Autodesk Inventor part; units mm, degrees
ref_plane "YZ Plane" through (0, 0, 0) normal (1, 0, 0) x (0, 1, 0)
ref_plane "XZ Plane" through (0, 0, 0) normal (0, 1, 0) x (-1, 0, 0)
ref_plane "XY Plane" through (0, 0, 0) normal (0, 0, 1) x (1, 0, 0)
sketch "Boceto1" plane through (0, 0, 0) normal (0, 1, 0) x (-1, 0, 0)
  line L0 (-97.5, 97.5) -> (97.5, 97.5)
  line L1 (97.5, 97.5) -> (97.5, -97.5)
  line L2 (97.5, -97.5) -> (-97.5, -97.5)
  line L3 (-97.5, -97.5) -> (-97.5, 97.5)
  line L4 (-97.5, 97.5) -> (97.5, -97.5) construction
  line L5 (97.5, 97.5) -> (-97.5, -97.5) construction
  point P0 (0, 0)
  dimension "d0" = 195
  dimension "d1" = 195
extrude "Extrusión1" add sketch "Boceto1" along normal mid plane 4.4
sketch "Boceto4" plane through (0, -2.2, 0) normal (0, -1, 0) x (1, 0, 0)
  line L0 (97.5, -97.5) -> (97.5, 97.5) construction
  line L1 (-97.5, 97.5) -> (-97.5, -97.5) construction
  line L2 (84.1, -93.1) -> (-84.1, -93.1)
  line L3 (-84.1, -93.1) -> (-84.1, -84.1)
  line L4 (-84.1, -84.1) -> (84.1, -84.1)
  line L5 (84.1, -84.1) -> (84.1, -93.1)
  line L6 (-97.5, -97.5) -> (97.5, -97.5) construction
  line L7 (93.1, -84.1) -> (84.1, -84.1)
  line L8 (84.1, -84.1) -> (84.1, 84.1)
  line L9 (84.1, 84.1) -> (93.1, 84.1)
  line L10 (93.1, 84.1) -> (93.1, -84.1)
  line L11 (0, -126.8945) -> (0, 107.949)
  line L12 (-84.1, -84.1) -> (-84.1, 84.1)
  line L13 (-84.1, 84.1) -> (-93.1, 84.1)
  line L14 (-93.1, 84.1) -> (-93.1, -84.1)
  line L15 (-93.1, -84.1) -> (-84.1, -84.1)
  line L16 (84.1, 84.1) -> (-84.1, 84.1)
  line L17 (84.1, 93.1) -> (-84.1, 93.1)
  line L18 (84.1, 84.1) -> (84.1, 93.1)
  line L19 (-84.1, 84.1) -> (-84.1, 93.1)
  point P0 (0, 0)
  point P1 (-84.1, -88.6)
  point P2 (88.6, -84.1)
  point P3 (84.1, -84.1)
  point P4 (84.1, -84.1)
  point P5 (84.1, -84.1)
  point P6 (84.1, -84.1)
  point P7 (-84.1, 84.1)
  point P8 (-84.1, 84.1)
  point P9 (-84.1, 84.1)
  point P10 (-84.1, 84.1)
  dimension "d20" = 4.4
  dimension "d21" = 9
  dimension "d22" = 13.4
  dimension "d23" = 13.4
  dimension "d24" = 4.4
  dimension "d25" = 9
  dimension "d26" = 13.4
  dimension "d30" = 9
extrude "Extrusión6" add sketch "Boceto4" along normal blind 9 contours L2 L11 L4 L5 | L2 L3 L4 L11 | L8 L9 L10 L7 | L16 L11 L17 L18 | L15 L14 L13 L12 | L16 L19 L17 L11
sketch "Boceto5" plane through (0, -11.2, 0) normal (0, -1, 0) x (1, 0, 0)
  line L0 (-84.1, -93.1) -> (84.1, -93.1) construction
  line L1 (93.1, -84.1) -> (93.1, 84.1) construction
  line L2 (-93.1, 84.1) -> (-93.1, -84.1) construction
  line L3 (84.1, 93.1) -> (-84.1, 93.1) construction
  line L4 (84.1, -93.1) -> (-84.1, -93.1)
  line L5 (-93.1, -84.1) -> (-93.1, 84.1)
  line L6 (-84.1, 93.1) -> (84.1, 93.1)
  line L7 (93.1, 84.1) -> (93.1, -84.1)
  line L8 (84.1, -93.1) -> (84.1, -84.1)
  line L9 (84.1, -84.1) -> (-84.1, -84.1) construction
  line L10 (84.1, -93.1) -> (84.1, -84.1)
  line L11 (84.1, -84.1) -> (93.1, -84.1)
  line L12 (93.1, 84.1) -> (84.1, 84.1)
  line L13 (84.1, 84.1) -> (84.1, 93.1)
  line L14 (-93.1, 84.1) -> (-84.1, 84.1)
  line L15 (-84.1, 84.1) -> (-84.1, 93.1)
  line L16 (-93.1, -84.1) -> (-84.1, -84.1)
  line L17 (-84.1, -93.1) -> (-84.1, -84.1)
  line L18 (-84.1, -84.1) -> (-93.1, -84.1)
  point P0 (0, 0)
extrude "Extrusión7" add sketch "Boceto5" along normal blind 1.65
sketch "Boceto6" plane through (0, -12.85, 0) normal (0, -1, 0) x (1, 0, 0)
  line L0 (-84.1, -84.1) -> (84.1, -84.1) construction
  line L1 (53.1, -84.1) -> (43.1, -84.1)
  line L2 (43.1, -84.1) -> (43.1, -64.1)
  line L3 (43.1, -64.1) -> (53.1, -64.1)
  line L4 (53.1, -64.1) -> (53.1, -84.1)
  line L5 (93.1, -84.1) -> (93.1, 84.1)
  line L6 (84.1, -84.1) -> (84.1, 84.1)
  line L7 (64.1, -53.1) -> (84.1, -53.1)
  line L8 (84.1, -53.1) -> (84.1, -43.1)
  line L9 (84.1, -43.1) -> (64.1, -43.1)
  line L10 (64.1, -43.1) -> (64.1, -53.1)
  line L11 (-84.1, -93.1) -> (84.1, -93.1)
  point P0 (0, 0)
  dimension "d35" = 40
  dimension "d36" = 10
  dimension "d37" = 20
  dimension "d38" = 40
  dimension "d39" = 10
  dimension "d40" = 20
extrude "Extrusión8" add sketch "Boceto6" along normal blind 15
sketch "Boceto7" plane through (43.1, -12.85, -84.1) normal (-1, 0, 0) x (0, 0, 1)
  line L0 (0, 0) -> (20, 0)
  line L1 (0, 0) -> (0, -15) construction
  line L2 (20, -15) -> (0, -15) construction
  line L3 (20, 0) -> (20, -15) construction
  line L4 (0, 0) -> (20, 0)
  circle A0 centre (10, -7.5) radius 3.85
  point P0 (84.1, 12.85)
  dimension "d43" = 7.7
extrude "Extrusión9" add sketch "Boceto7" along normal blind 4
sketch "Boceto8" plane through (39.1, -20.35, -74.1) normal (-1, 0, 0) x (0, 0, 1)
  circle A0 centre (0, 0) radius 3.85
  circle A1 centre (0, 0) radius 7.25
  point P0 (74.1, 20.35)
  dimension "d46" = 14.5
extrude "Extrusión10" add sketch "Boceto8" along normal up to surface (39.1 mm away)
sketch "Boceto10" plane through (39.1, -20.35, -74.1) normal (-1, 0, 0) x (0, 0, 1)
  circle A0 centre (0, 0) radius 3.85
  point P0 (74.1, 20.35)
extrude "Extrusión11" add sketch "Boceto10" along normal up to surface (39.1 mm away)
mirror "Simetría4" about plane through (0, 0, 0) normal (1, 0, 0) of "Extrusión9", "Extrusión10", "Extrusión11", "Extrusión8"
sketch "Boceto11" plane through (-84.1, -27.85, -53.1) normal (0, -1, 0) x (1, 0, 0)
  line L0 (20, 0) -> (0, 0)
  line L1 (20, 10) -> (20, 0)
  line L2 (0, 10) -> (20, 10)
  line L3 (0, 0) -> (0, 10)
  point P0 (84.1, 53.1)
extrude "Extrusión12" cut sketch "Boceto11" against normal up to surface (15 mm away)
sketch "Boceto12" plane through (64.1, -12.85, -43.1) normal (0, 0, 1) x (1, 0, 0)
  line L0 (0, 0) -> (20, 0)
  line L1 (0, 0) -> (0, -15)
  line L2 (20, -15) -> (0, -15)
  line L3 (20, 0) -> (20, -15)
  circle A0 centre (10, -7.5) radius 3.85
  point P0 (-64.1, 12.85)
  dimension "d53" = 7.7
extrude "Extrusión13" add sketch "Boceto12" along normal blind 4 contours A0
sketch "Boceto13" plane through (74.1, -20.35, -39.1) normal (0, 0, 1) x (1, 0, 0)
  circle A0 centre (0, 0) radius 3.85
  circle A1 centre (0, 0) radius 7.25
  point P0 (-74.1, 20.35)
  dimension "d56" = 14.5
extrude "Extrusión14" add sketch "Boceto13" along normal up to surface (39.1 mm away)
sketch "Boceto14" plane through (74.1, -20.35, -39.1) normal (0, 0, 1) x (1, 0, 0)
  circle A0 centre (0, 0) radius 3.85
  point P0 (-74.1, 20.35)
extrude "Extrusión15" add sketch "Boceto14" along normal up to surface (39.1 mm away)
mirror "Simetría5" about plane through (0, 0, 0) normal (0, 0, 1) of "Extrusión15", "Extrusión14", "Extrusión13", "Extrusión12", "Extrusión8"
sketch "Boceto15" plane through (43.1, -27.85, 64.1) normal (0, -1, 0) x (1, 0, 0)
  line L0 (10, 0) -> (0, 0)
  line L1 (10, 20) -> (10, 0)
  line L2 (0, 20) -> (10, 20)
  line L3 (0, 0) -> (0, 20)
  point P0 (-43.1, -64.1)
extrude "Extrusión16" cut sketch "Boceto15" against normal up to surface (15 mm away)
sketch "Boceto16" plane through (0, -12.85, 0) normal (0, -1, 0) x (1, 0, 0)
  line L0 (81.35, 39.1) -> (66.85, 39.1) construction
  line L1 (81.35, -39.1) -> (66.85, -39.1) construction
  line L2 (81.35, -39.1) -> (81.35, 39.1) construction
  line L3 (66.85, -39.1) -> (66.85, 39.1) construction
  line L4 (81.35, -39.1) -> (66.85, -39.1) construction
  line L5 (81.35, 39.1) -> (66.85, 39.1) construction
  line L6 (-39.1, -66.85) -> (-39.1, -81.35)
  line L7 (39.1, -66.85) -> (39.1, -81.35)
  line L8 (-81.35, -44.335) -> (-66.85, -44.335)
  line L9 (-66.85, -44.335) -> (-66.85, 44.335)
  line L10 (-66.85, 44.335) -> (-81.35, 44.335)
  line L11 (-81.35, 44.335) -> (-81.35, -44.335)
  line L12 (-93.1, 84.1) -> (-93.1, -84.1) construction
  line L13 (84.1, 93.1) -> (-84.1, 93.1) construction
  line L14 (-44.335, 81.35) -> (-44.335, 66.85)
  line L15 (-44.335, 66.85) -> (44.335, 66.85)
  line L16 (44.335, 66.85) -> (44.335, 81.35)
  line L17 (44.335, 81.35) -> (-44.335, 81.35)
  point P0 (0, 0)
  dimension "d84" = 11.75
  dimension "d85" = 14.5
  dimension "d86" = 88.67
  dimension "d87" = 48.765
  dimension "d88" = 14.5
  dimension "d89" = 88.67
  dimension "d90" = 48.765
  dimension "d91" = 11.75
sketch "Boceto17" plane through (0, -12.85, 0) normal (0, -1, 0) x (1, 0, 0)
  line L0 (50.85, 50.85) -> (-50.85, 50.85) construction
  line L1 (-50.85, 50.85) -> (-50.85, -50.85) construction
  line L2 (-50.85, -50.85) -> (50.85, -50.85) construction
  line L3 (50.85, -50.85) -> (50.85, 50.85) construction
  line L4 (50.85, 50.85) -> (-50.85, -50.85) construction
  line L5 (-50.85, 50.85) -> (50.85, -50.85) construction
  circle A0 centre (40.85, 40.85) radius 2.5
  circle A1 centre (-40.85, 40.85) radius 2.5
  line L6 (101.7, 0) -> (-109.1959, 0)
  circle A2 centre (40.85, -40.85) radius 2.5
  circle A3 centre (-40.85, -40.85) radius 2.5
  point P0 (0, 0)
  dimension "d67" = 101.7
  dimension "d68" = 101.7
  dimension "d69" = 5
  dimension "d70" = 10
  dimension "d71" = 10
  dimension "d72" = 10
  dimension "d73" = 10
  dimension "d94" = 5
  dimension "d95" = 5
extrude "Extrusión19" add sketch "Boceto17" along normal blind 100.95
sketch "Boceto18" plane through (0, -12.85, 0) normal (0, -1, 0) x (1, 0, 0)
  line L0 (84.1, 93.1) -> (-84.1, 93.1)
  line L1 (-84.1, 93.1) -> (-84.1, 84.1)
  line L2 (-84.1, 84.1) -> (-93.1, 84.1)
  line L3 (-93.1, 84.1) -> (-93.1, -84.1)
  line L4 (-93.1, -84.1) -> (-84.1, -84.1)
  line L5 (-84.1, -84.1) -> (-84.1, -93.1)
  line L6 (-84.1, -93.1) -> (84.1, -93.1)
  line L7 (84.1, -93.1) -> (84.1, -84.1)
  line L8 (93.1, -84.1) -> (93.1, 84.1)
  line L9 (84.1, -84.1) -> (93.1, -84.1)
  line L10 (93.1, 84.1) -> (84.1, 84.1)
  line L11 (84.1, 84.1) -> (84.1, 93.1)
  line L12 (-81.0533, 90.0533) -> (81.0533, 90.0533)
  line L13 (81.0533, 90.0533) -> (81.0533, 81.0533)
  line L14 (81.0533, 81.0533) -> (90.0533, 81.0533)
  line L15 (90.0533, 81.0533) -> (90.0533, -81.0533)
  line L16 (90.0533, -81.0533) -> (81.0533, -81.0533)
  line L17 (81.0533, -81.0533) -> (81.0533, -90.0533)
  line L18 (81.0533, -90.0533) -> (-81.0533, -90.0533)
  line L19 (-81.0533, -90.0533) -> (-81.0533, -81.0533)
  line L20 (-81.0533, -81.0533) -> (-90.0533, -81.0533)
  line L21 (-90.0533, -81.0533) -> (-90.0533, 81.0533)
  line L22 (-90.0533, 81.0533) -> (-81.0533, 81.0533)
  line L23 (-81.0533, 81.0533) -> (-81.0533, 90.0533)
  point P0 (0, 0)
extrude "Extrusión20" cut sketch "Boceto18" against normal blind 1.65
sketch "Boceto19" plane through (0, -12.85, 0) normal (0, -1, 0) x (1, 0, 0)
  circle A0 centre (-40.85, -40.85) radius 2.5 construction
  circle A1 centre (-40.85, -40.85) radius 2.5 construction
  circle A2 centre (-40.85, -40.85) radius 4
  line L0 (-66.85, -39.1) -> (-66.85, 39.1)
  circle A3 centre (-40.85, 40.85) radius 2.5 construction
  circle A4 centre (-40.85, 40.85) radius 4
  line L1 (0, -105.6023) -> (0, 128.9456)
  circle A5 centre (40.85, -40.85) radius 2.5 construction
  circle A6 centre (40.85, -40.85) radius 2.5 construction
  circle A7 centre (40.85, -40.85) radius 4
  circle A8 centre (40.85, 40.85) radius 2.5 construction
  circle A9 centre (40.85, 40.85) radius 4
  circle A10 centre (40.85, -40.85) radius 2.5 construction
  circle A11 centre (40.85, -40.85) radius 2.5 construction
  circle A12 centre (40.85, 40.85) radius 2.5 construction
  circle A13 centre (-40.85, 40.85) radius 2.5 construction
  point P0 (0, 0)
  dimension "d78" = 8
  dimension "d79" = 8
extrude "Extrusión21" add sketch "Boceto19" along normal blind 19.1
extrude "Extrusión22" add sketch "Boceto16" along normal blind 15
properties part number "Acrilico_Bottom"
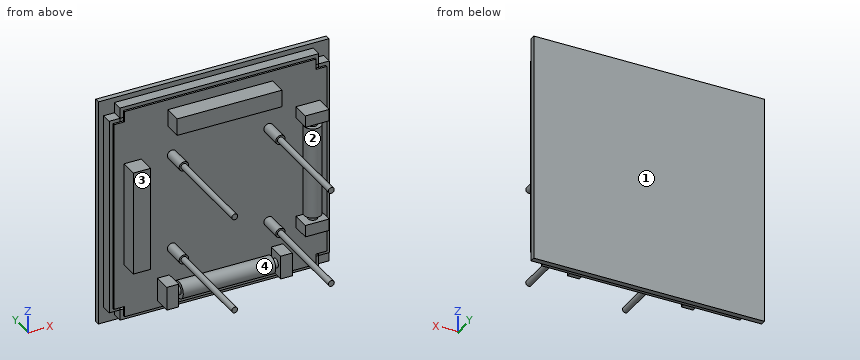
Here's how the part is built. I have some questions about the finished solid (model axes, mm). Face numbers are marked on the shaded views. Give positions to 0.01 mm unless a question says otherwise; leave off trailing zeros. Order: outer loops, then holes, each group sorted by start corner. A loop starts at its lowest first (then second) coordinate and runs counter-clockwise, first axis right, second up. Notation, with made-up numbers: (88, -18.75) -> (102, -18.75) arc R28 cw to (102, 0.25) -> close; hole circle Ø2 at (-8, 21.25). An arc over 180 degrees is marked (long way). Use a Markdown table: item, result. Add a question column.
Item 1: If we mould it in two halves opening along Y, with no side actions, what happens to the marked faces 1, 2, 3 and 4? For each: pulls with the +Y half, pulls with the -Y half, needs draft (parallel to the pull), parting line crosses it, or undercut.
Item 2: Imagine slicing it at D-D on y = -78.5. Please give me the cut outline in (x, z).
Item 3: I need wall thicknesses on line 1 (Y direction, x = -24, z = 77); line 2 (Y direction, x = -8, z = 48.5); line 3 (X direction, y = -14.5, z = 41.5). Which ranges of each line are inside material? Lowest first, please.
Item 4: Will these pins go through, and if not, where does the flat tip stop? pin 1 (8 mm diameter, centred on x = 75, z = -48, fed in from -Y); pin 2 (4 mm diameter, centred on x = 43.5, y = -80.5, fed in from +Z); pin 3 (4.5 mm diameter, centred on x = 71, y = -21, fed in from +Z).
Item 5: Imagine slicing it at B-B on z = -26. Please give me the cut outline in (x, y), plus the area to 3 significant figures.
Item 6: Imagine slicing it at C-C on z = 72. Please give me the cut outline in (x, y) (3 decimals), plus the area to 3 significant figures.
Item 7: Imagine slicing it at A-A on x = -4.5. Please give me the cut outline in (y, z), plus the area to 3 significant figures.
Data:
| question | item | result |
|---|---|---|
| 1 | face 1 | pulls with the +Y half |
| 1 | face 2 | undercut |
| 1 | face 3 | pulls with the -Y half |
| 1 | face 4 | undercut |
| 2 | outline | circle Ø5 at (-40.85, -40.85); circle Ø5 at (-40.85, 40.85); circle Ø5 at (40.85, -40.85); circle Ø5 at (40.85, 40.85) |
| 3 | line 1 | y = -27.85 to -11.2, -2.2 to 2.2 |
| 3 | line 2 | y = -12.85 to -11.2, -2.2 to 2.2 |
| 3 | line 3 | x = -81.35 to -66.85, -44.8 to -36.9, 36.9 to 44.8 |
| 4 | pin 1 | stops at y = -27.85 |
| 4 | pin 2 | stops at z = 43.26 |
| 4 | pin 3 | stops at z = 53.1 |
| 5 | outline | (-97.5, -2.2) -> (-93.1, -2.2) -> (-93.1, -11.2) -> (-90.05, -11.2) -> (-90.05, -12.85) -> (-81.35, -12.85) -> (-81.35, -27.85) -> (-66.85, -27.85) -> (-66.85, -12.85) -> (90.05, -12.85) -> (90.05, -11.2) -> (93.1, -11.2) -> (93.1, -2.2) -> (97.5, -2.2) -> (97.5, 2.2) -> (-97.5, 2.2) -> close; circle Ø14.5 at (74.1, -20.35); hole (-84.1, -11.2) -> (84.1, -11.2) -> (84.1, -2.2) -> (-84.1, -2.2) -> close |
| 5 | area | 1,700 mm² |
| 6 | outline | (-97.5, -2.2) -> (-93.1, -2.2) -> (-93.1, -11.2) -> (-90.053, -11.2) -> (-90.053, -12.85) -> (-44.335, -12.85) -> (-44.335, -27.85) -> (44.335, -27.85) -> (44.335, -12.85) -> (90.053, -12.85) -> (90.053, -11.2) -> (93.1, -11.2) -> (93.1, -2.2) -> (97.5, -2.2) -> (97.5, 2.2) -> (-97.5, 2.2) -> close; hole (-84.1, -11.2) -> (84.1, -11.2) -> (84.1, -2.2) -> (-84.1, -2.2) -> close |
| 6 | area | 2,650 mm² |
| 7 | outline | (-27.85, 66.85) -> (-12.85, 66.85) -> (-12.85, -90.05) -> (-11.2, -90.05) -> (-11.2, -93.1) -> (-2.2, -93.1) -> (-2.2, -97.5) -> (2.2, -97.5) -> (2.2, 97.5) -> (-2.2, 97.5) -> (-2.2, 93.1) -> (-11.2, 93.1) -> (-11.2, 90.05) -> (-12.85, 90.05) -> (-12.85, 81.35) -> (-27.85, 81.35) -> close; circle Ø14.5 at (-20.35, -74.1); hole (-11.2, -84.1) -> (-2.2, -84.1) -> (-2.2, 84.1) -> (-11.2, 84.1) -> close |
| 7 | area | 1,700 mm² |
